Job drawing, mm, ordinate dimensions from the low corner. One solid piece. Give positions to 0.01 mm unless a question says otherwise; leave off trailing zeros. Loops run counter-clockwise (first coordinate to the right, second up) from the corner with the lowest first, then second, coordinate; pieces in that order, holes last. Notation, with made-up numbers: (44, -36) - (51, -36) arc R32 cw to (51, -1) - close; hole circle Ø1 at (-2, 78). An arc over 180 degrees is marked (long way). Use a Markdown table: item, result.
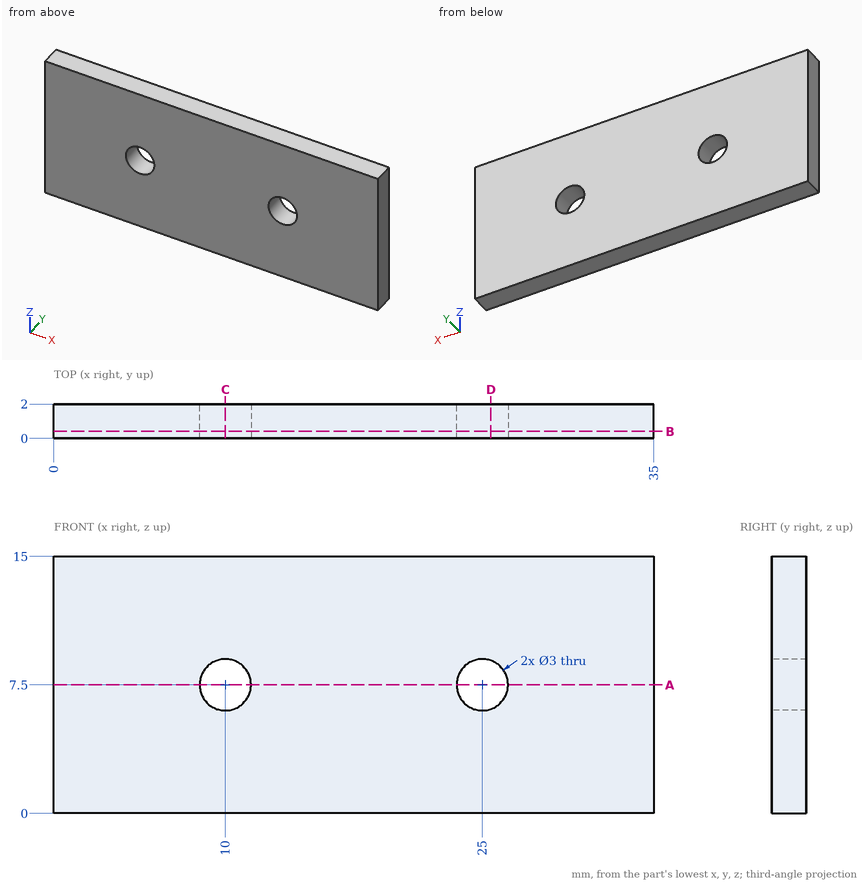
(1) Slice it at B-B, the plane y = 0.4. Write the cut outline in (x, z).
Computed:
| item | result |
|---|---|
| outline | (0, 0) - (35, 0) - (35, 15) - (0, 15) - close; hole circle Ø3 at (10, 7.5); hole circle Ø3 at (25, 7.5) |
(2) Slice it at A-A, the plane z = 7.5. Write the cut outline in (x, y).
Computed:
| item | result |
|---|---|
| outline | (0, 0) - (8.5, 0) - (8.5, 2) - (0, 2) - close; (11.5, 0) - (23.5, 0) - (23.5, 2) - (11.5, 2) - close; (26.5, 0) - (35, 0) - (35, 2) - (26.5, 2) - close |
(3) Slice it at C-C, the plane x = 10. Write the cut outline in (y, z).
Computed:
| item | result |
|---|---|
| outline | (0, 0) - (2, 0) - (2, 6) - (0, 6) - close; (0, 9) - (2, 9) - (2, 15) - (0, 15) - close |
(4) Slice it at D-D, the plane x = 25.5. Write the cut outline in (y, z).
Computed:
| item | result |
|---|---|
| outline | (0, 0) - (2, 0) - (2, 6.09) - (0, 6.09) - close; (0, 8.91) - (2, 8.91) - (2, 15) - (0, 15) - close |
(5) Drill centre lines: probe 1 along X at (y, z) = (1.55, 7.5); probe 2 along Z at (x, y) = (25, 0.7); probe 3 along Z at (x, y) = (25.5, 0.85). Where is each one in solid material? Low to high. Write a range as [from, to].
Computed:
| item | result |
|---|---|
| probe 1 | [0, 8.5], [11.5, 23.5], [26.5, 35] |
| probe 2 | [0, 6], [9, 15] |
| probe 3 | [0, 6.09], [8.91, 15] |
